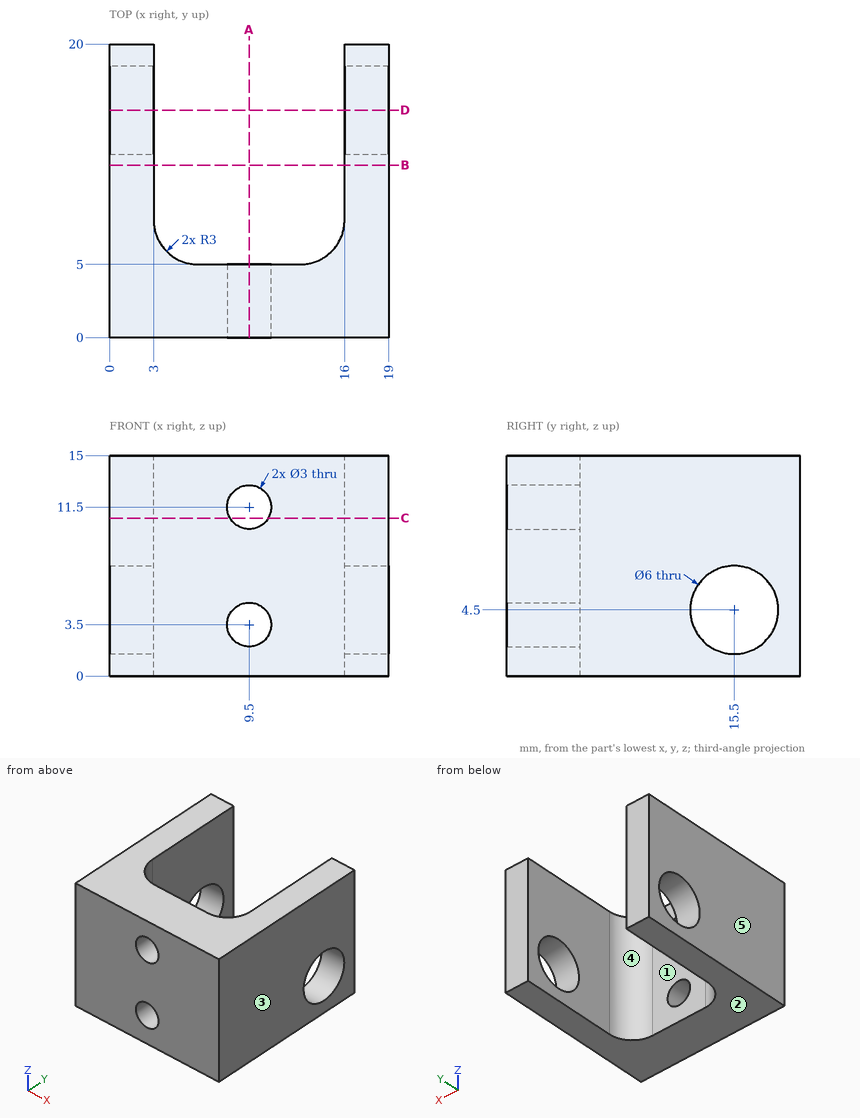
Drawing for the job (mm, zero at the part's lowest x, y, z). A direction names the side the tool comes from. Round coordinates to 2 decimals unless told otherwise and drop trailing zeros. Write each loop counter-clockwise with the first axis right and the second up, starting at its lowest first coordinate (ties: lowest second). Pieces come first, ordered by that corner, then holes. Notation, with made-up numbers: (-24.75, -19) - (17.25, -19) arc R22 cw to (17.25, -7) - close; hole circle Ø2 at (0, 41.25). An arc over 180 degrees is marked (long way). Use CSV: the item, a comma, the result in double quotes.
(1) Wall check: line 1 (Z direction, x = 18.15, y = 15.5); line 2 (X direction, y = 2.3, z = 11.5); line 3 (X direction, y = 16.5, z = 1.25). Give the ranges that are in metal, low to high.
Response:
line 1,"0 to 1.5, 7.5 to 15"
line 2,"0 to 8, 11 to 19"
line 3,"0 to 3, 16 to 19"
(2) Band-saw the part on B-B (y = 11.75). Write the cut outline in (x, z).
Response:
outline,"(0, 0) - (3, 0) - (3, 15) - (0, 15) - close; (16, 0) - (19, 0) - (19, 15) - (16, 15) - close"
(3) Band-saw the part on C-C (z = 10.75). Write the cut outline in (x, y).
Response:
outline,"(0, 0) - (8.2, 0) - (8.2, 5) - (6, 5) arc R3 cw to (3, 8) - (3, 20) - (0, 20) - close; (10.8, 0) - (19, 0) - (19, 20) - (16, 20) - (16, 8) arc R3 cw to (13, 5) - (10.8, 5) - close"
(4) Band-saw the part on D-D (y = 15.5). Write the cut outline in (x, z), plus the area to 3 significant figures.
Response:
outline,"(0, 0) - (3, 0) - (3, 1.5) - (0, 1.5) - close; (0, 7.5) - (3, 7.5) - (3, 15) - (0, 15) - close; (16, 0) - (19, 0) - (19, 1.5) - (16, 1.5) - close; (16, 7.5) - (19, 7.5) - (19, 15) - (16, 15) - close"
area,"54.0 mm²"
(5) 3-axis set-ups, long thin cutter, end or side, ignore diameter. For the marked faces 4 and 5: which of +Z, -Z, +X, -X, +Y, -Y reach the whole face in a straight line?
Response:
face 4,"+Z, -Z, +Y"
face 5,"+Z, -Z, -X, +Y, -Y"
(6) Pin check, flat tips, straight feed: P1, Ø5, axis at x = 9.5, z = 3.5, coming from the +Y side; P2, Ø8, axis at y = 15.5, z = 4.5, coming from the -X side; P3, Ø8, axis at x = 11.5, z = 9.5, coming from the +Y side. Stop position of each tip, or through.
Response:
P1,"y = 5"
P2,"x = 0"
P3,"y = 6.34"
(7) Band-saw the part on A-A (x = 9.5). Write the cut outline in (y, z), plus the area to 3 significant figures.
Response:
outline,"(0, 0) - (5, 0) - (5, 2) - (0, 2) - close; (0, 5) - (5, 5) - (5, 10) - (0, 10) - close; (0, 13) - (5, 13) - (5, 15) - (0, 15) - close"
area,"45.0 mm²"
(8) Mould opens along X. For the marked faces 1, 2 and 3 say: pulls with the +X half, pulls with the -X half, needs draft (parallel to the pull), parting line crosses it, or undercut.
Response:
face 1,"undercut"
face 2,"needs draft"
face 3,"pulls with the +X half"
